Verification items for the finished model (mm, model axes). Face numbers are marked on the shaded views. A direction names the side the tool comes from. Round coordinates to 2 decimals unless told otherwise and drop trailing zeros. Write each loop counter-clockwise with the first axis right and the second up, starting at its lowest first coordinate (ties: lowest second). Pieces come first, ordered by that corner, then holes. Notation, with made-up numbers: M 18,55.5 L 59,55.5 A35 ccw 59,92.5 Z; hole C 7,72.5 d4. An arc over 180 degrees is marked long. Use a Markdown table: item, result. Add a question column.
from build123d import *

# Parameters (mm, degrees)
CHAMFER_1_SIZE = 0.2
CHAMFER_2_SIZE = 0.2
CHAMFER_3_SIZE = 0.2
CHAMFER_4_SIZE = 0.2


with BuildPart() as part:
    # Эскиз1 → Повернуть1 (revolve)
    with BuildSketch(Plane.XY):
        Polygon((-30.2, 0), (-30.2, 264.999961118), (-28.25, 264.999961118), (-28.25, 229.999961118), (-28, 229.999961118), (-28, 25), (-28.25, 25), (-28.25, 0), align=None)
    revolve(axis=Axis((0, 0, 0), (0, 1, 0)))

    # Фаска1
    chamfer_1_edges = [part.edges().sort_by_distance(p)[0] for p in [
        (30.2, 264.999961118, 0),
    ]]
    chamfer(chamfer_1_edges, length=CHAMFER_1_SIZE)

    # Фаска2
    chamfer_2_edges = [part.edges().sort_by_distance(p)[0] for p in [
        (28.25, 264.999961118, 0),
        (28.25, 229.999961118, 0),
    ]]
    chamfer(chamfer_2_edges, length=CHAMFER_2_SIZE)

    # Фаска3
    chamfer_3_edges = [part.edges().sort_by_distance(p)[0] for p in [
        (30.2, 0, 0),
    ]]
    chamfer(chamfer_3_edges, length=CHAMFER_3_SIZE)

    # Фаска4
    chamfer_4_edges = [part.edges().sort_by_distance(p)[0] for p in [
        (28.25, 0, 0),
    ]]
    chamfer(chamfer_4_edges, length=CHAMFER_4_SIZE)


solid = part.part
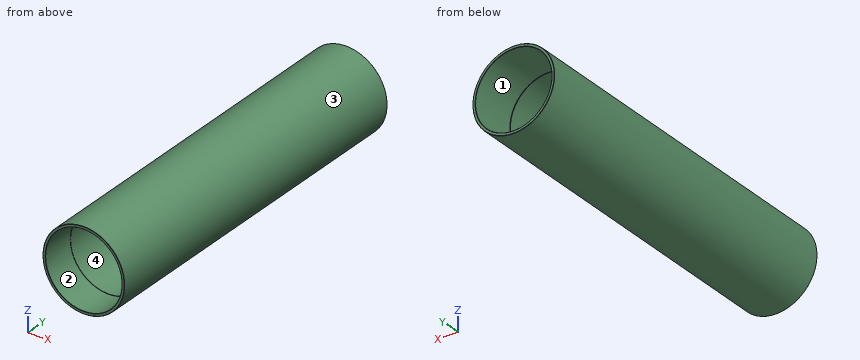
1. Cross-section at A-A on z = 0. Enter the section's corners in (x, y), plus the area to 3 significant figures.
2. Cross-section at B-B on x = 0. Enter the section's corners in (y, z), plus the area to 3 significant figures.
3. Scan lines: line 1 along Z through (x, y) = (0, 93); line 2 along Z through (x, y) = (0, 15.5); line 3 along X through (y, z) = (90, -22). Record each from-to range of solid material in increasing order. Write a range as from..to.
4. Release check for a two-part mould opening along Z. For the marked faces 3 and 4 record: +Z half, -Z half, draft (parallel to the pull), parting line (faces both ways), or undercut.
5. Depth check by flat-ended pin: pin 1 Ø2 at (y, z) = (217.5, -7) entering from -X; pin 2 Ø1.5 at (x, y) = (16.5, 233.5) entering from +Z; pin 3 Ø2 at (x, y) = (0.5, 185.5) entering from -Z; pin 4 Ø17 at (x, z) = (2.5, 12) entering from +Y. Enter the tip coordinate at first touch or a pass-through.
6. Cross-section at C-C on y = 68. Enter the section's corners in (x, z).
7. Access from +Z, -Z, +X, -X, +Y, -Y to the whole of each face (thin tool, end or side, straight path). Record for the marked faces 1 and 2.
Answer:
| question | item | result |
|---|---|---|
| 1 | outline | M -30.2,0.2 L -30,0 L -28.45,0 L -28.25,0.2 L -28.25,25 L -28,25 L -28,230 L -28.05,230 L -28.25,230.2 L -28.25,264.8 L -28.45,265 L -30,265 L -30.2,264.8 Z; M 28,25 L 28.25,25 L 28.25,0.2 L 28.45,0 L 30,0 L 30.2,0.2 L 30.2,264.8 L 30,265 L 28.45,265 L 28.25,264.8 L 28.25,230.2 L 28.05,230 L 28,230 Z |
| 1 | area | 1,140 mm^2 |
| 2 | outline | M 0,-30 L 0.2,-30.2 L 264.8,-30.2 L 265,-30 L 265,-28.45 L 264.8,-28.25 L 230.2,-28.25 L 230,-28.05 L 230,-28 L 25,-28 L 25,-28.25 L 0.2,-28.25 L 0,-28.45 Z; M 0,28.45 L 0.2,28.25 L 25,28.25 L 25,28 L 230,28 L 230,28.05 L 230.2,28.25 L 264.8,28.25 L 265,28.45 L 265,30 L 264.8,30.2 L 0.2,30.2 L 0,30 Z |
| 2 | area | 1,140 mm^2 |
| 3 | line 1 | z = -30.2..-28, 28..30.2 |
| 3 | line 2 | z = -30.2..-28.25, 28.25..30.2 |
| 3 | line 3 | x = -20.69..-17.32, 17.32..20.69 |
| 4 | face 3 | parting line |
| 4 | face 4 | undercut |
| 5 | pin 1 | stops at x = -29.6 |
| 5 | pin 2 | stops at z = 25.77 |
| 5 | pin 3 | stops at z = -30.2 |
| 5 | pin 4 | passes through |
| 6 | outline | C 0,0 d60.4; hole C 0,0 d56 |
| 7 | face 1 | +Y |
| 7 | face 2 | -Y |
